Autodesk Inventor part; units mm, degrees
ref_plane "YZ Plane" through (0, 0, 0) normal (1, 0, 0) x (0, 1, 0)
ref_plane "XZ Plane" through (0, 0, 0) normal (0, 1, 0) x (-1, 0, 0)
ref_plane "XY Plane" through (0, 0, 0) normal (0, 0, 1) x (1, 0, 0)
sketch "Sketch1" plane through (0, 0, 0) normal (0, 0, 1) x (1, 0, 0)
  arc A0 (2.8466, -52.6517) -> (4.2608, -52.0659) centre (2.8466, -50.6517) ccw
  line L0 (4.2608, -52.0659) -> (25.703, -30.6237)
  arc A1 (25.703, -30.6237) -> (26.2888, -29.2095) centre (24.2888, -29.2095) ccw
  line L1 (26.2888, -29.2095) -> (26.2888, 17.012)
  arc A2 (26.2888, 17.012) -> (25.8127, 18.3073) centre (24.2888, 17.012) ccw
  line L2 (25.8127, 18.3073) -> (13.9072, 32.3139)
  arc A3 (13.9072, 32.3139) -> (13.1317, 32.8733) centre (12.3833, 31.0186) ccw
  arc A4 (-11.6683, 32.8733) -> (-12.4438, 32.3139) centre (-10.9199, 31.0186) ccw
  line L3 (-12.4438, 32.3139) -> (-20.1922, 23.1981)
  arc A5 (-20.1922, 23.1981) -> (-20.6683, 21.9028) centre (-18.6683, 21.9028) ccw
  line L4 (-20.6683, 21.9028) -> (-20.6683, 4.4299)
  line L5 (-20.6683, 4.4299) -> (-27.2, -2.1017)
  arc A6 (-139.695, -52.3056) -> (-138.5704, -52.6517) centre (-138.5704, -50.6517) ccw
  arc A7 (-138.5704, -2.1017) -> (-139.695, -2.4479) centre (-138.5704, -4.1017) ccw
  line L6 (-139.695, -2.4479) -> (-143.4444, -4.9975)
  arc A8 (-143.4444, -4.9975) -> (-143.4828, -5.023) centre (-142.3581, -6.6767) ccw
  line L7 (-143.4828, -5.023) -> (-149.2963, -8.9767)
  line L8 (-149.2963, -8.9767) -> (-151.4209, -10.4215)
  arc A9 (-151.4209, -10.4215) -> (-152.2963, -12.0753) centre (-150.2963, -12.0753) ccw
  line L9 (-152.2963, -12.0753) -> (-152.2963, -12.6767)
  line L10 (-152.2963, -42.0767) -> (-152.2963, -42.6781)
  arc A10 (-152.2963, -42.6781) -> (-151.4209, -44.332) centre (-150.2963, -42.6781) ccw
  line L11 (-151.4209, -44.332) -> (-139.695, -52.3056)
  arc A11 (-5.1284, 30.1824) -> (-4.7861, 30.3893) centre (0.7317, 20.8733) ccw
  arc A12 (-148.0905, -39.6176) -> (-148.4375, -39.4185) centre (-141.2963, -27.3767) ccw
  line L12 (-11.6683, 32.8733) -> (13.1317, 32.8733)
  line L13 (-152.2963, -12.6767) -> (-152.2963, -18.7165)
  line L14 (-152.2963, -36.037) -> (-152.2963, -42.0767)
  line L15 (2.8466, -52.6517) -> (-138.5704, -52.6517)
  line L16 (-138.5704, -2.1017) -> (-27.2, -2.1017)
  circle A13 centre (0.7317, 20.8733) radius 11
  circle A14 centre (-141.2963, -27.3767) radius 14
extrude "Extrusion1" add sketch "Sketch1" along normal mid plane 36.75 contours L15 A6 L11 A10 L10 L14 A12 A14 L13 L9 A9 L8 L7 A8 L6 A7 L16 L5 L4 A5 L3 A4 L12 A3 L2 A2 L1 A1 L0 A0
extrude "Extrusion2" add sketch "Sketch1" along normal mid plane 47 contours A12 A14
extrude "Extrusion3" add sketch "Sketch1" along normal mid plane 41 contours A13 A11
properties part number "Bicep"
Verification items for the finished model (mm, model axes). A direction names the side the tool comes from. Round coordinates to 2 decimals unless told otherwise and drop trailing zeros. Write each loop counter-clockwise with the first axis right and the second up, starting at its lowest first coordinate (ties: lowest second). Pieces come first, ordered by that corner, then holes. Notation, with made-up numbers: (70, -22) -> (99, -22) arc R10 ccw to (99, -11) -> close; hole circle Ø11 at (21.5, 87.25). An arc over 180 degrees is marked (long way). Write each question's results on one line, items separated by ' | '. Start each with the question number.
1. Cross-section at D-D (x = -85). Enter the section's corners in (y, z) (3 decimals).
2. Cross-section at A-A (x = -132.5). Enter the section's corners in (y, z) (3 decimals).
3. Set-up check for faces 1 (the cylindrical face through (-155.288, -27.893, -0.329)), 2 (the flat face through (-152.296, -39, 0)), 3 (the flat face through (-84, -2.102, 0)): record each of +Z, -Z, +X, -X, +Y, -Y from which the full face is reachable in a straight line by a thin tool's end or side.
4. Depth check by flat-ended pin: P1, Ø4, axis at x = -122.5, y = -14, coming from the +Z side (3 decimals); P2, Ø6, axis at x = 5.5, y = -24.5, coming from the -Z side (3 decimals); P3, Ø2, axis at y = -40.5, z = -5.5, coming from the -X side. Enter the tip coordinate at first touch or a pass-through.
5. Material ranges on probe 1 along X at (y, z) = (4.5, 13.5); probe 2 along Z at (x, y) = (10.5, -12) (3 decimals); probe 3 along X at (y, z) = (-5, 7), recorded low to high. Write a range as from..to.
6. Cross-section at B-B (y = -16.5). Enter the section's corners in (x, z) (3 decimals), then the cut area to 3 significant figures.
Solutions:
1) outline: (-52.652, -18.375) -> (-2.102, -18.375) -> (-2.102, 18.375) -> (-52.652, 18.375) -> close
2) outline: (-52.652, -18.375) -> (-38.267, -18.375) -> (-38.267, -23.5) -> (-16.485, -23.5) -> (-16.485, -18.375) -> (-2.102, -18.375) -> (-2.102, 18.375) -> (-16.485, 18.375) -> (-16.485, 23.5) -> (-38.267, 23.5) -> (-38.267, 18.375) -> (-52.652, 18.375) -> close
3) face 1: none | face 2: +Z, -Z, -X, -Y | face 3: +Z, -Z, -X, +Y
4) P1: stops at z = 18.375 | P2: stops at z = -18.375 | P3: stops at x = -152.3
5) probe 1: x = -20.67..26.29 | probe 2: z = -18.375..18.375 | probe 3: x = -143.45..26.29
6) outline: (-152.296, -18.375) -> (-150.113, -18.375) -> (-150.113, -23.5) -> (-132.482, -23.5) -> (-132.482, -18.375) -> (26.289, -18.375) -> (26.289, 18.375) -> (-132.482, 18.375) -> (-132.482, 23.5) -> (-150.113, 23.5) -> (-150.113, 18.375) -> (-152.296, 18.375) -> close | area: 6,740 mm2
